Input: dimensioned drawing with shaded views. Units: mm. Origin: part minimum x, y, z. A direction names the side the tool comes from. Round coordinates to 2 decimals unless told otherwise and drop trailing zeros. Write each loop counter-clockwise with the first axis right and the second up, starting at its lowest first coordinate (ties: lowest second). Pieces come first, ordered by that corner, then holes. Notation, with made-up numbers: (68.25, 88) -> (100.25, 88) arc R18 cw to (100.25, 99) -> close; hole circle Ø10 at (43.25, 73). An arc over 180 degrees is marked (long way). One line per item, written item: value. Start each with the question number.
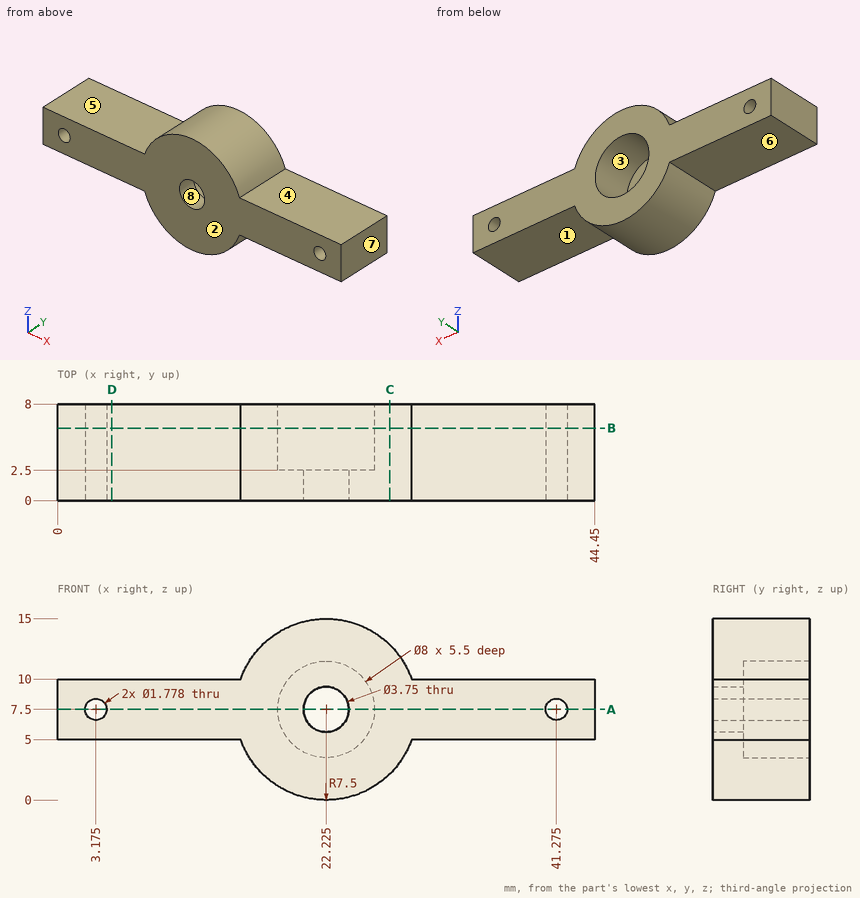
(1) Line query: probe 1 along X at (y, z) = (5.45, 7.5) (3 decimals); probe 2 along X at (y, z) = (1.5, 7.75); probe 3 along Z at (x, y) = (40, 6.5). Output: solid intervals per line, ascending.
(2) Section query D-D (x = 4.5). Output: boundary loops of the cut face in (y, z).
(3) Pull-direction query (X, two-part tool) for the marked faces 6, 7 and 8; classes: pulls with the +X half, pulls with the -X half, needs draft (parallel to the pull), parting line crosses it, or undercut.
(4) Section query B-B (y = 6). Output: boundary loops of the cut face in (x, z) (3 decimals), and give its area (3 significant figures).
(5) Section query C-C (x = 27.5). Output: boundary loops of the cut face in (y, z).
(6) Section query A-A (z = 7.5). Output: boundary loops of the cut face in (x, y) (3 decimals).
(7) Set-up query: the marked faces 1, 2, 3, 4 and 5. Return all of +Z, -Z, +X, -X, +Y, -Y with unobstructed straight access to the full face (end or side cutting, diameter ignored); none if empty.
(8) Pin query (flat end, axial travel): pin 1 (5 mm diameter, centred on x = 21, z = 8, fed in from +Y); pin 2 (2.5 mm diameter, centred on x = 8.5, y = 3, fed in from -Z); pin 3 (1.6 mm diameter, centred on x = 41.275, z = 7.5, fed in from +Y); pin 4 (4 mm diameter, centred on x = 5, y = 5.5, fed in from +Z). Return the tip coordinate at first contact, or that it passes through.
Results list:
1. probe 1: x = 0 to 2.286, 4.064 to 18.225, 26.225 to 40.386, 42.164 to 44.45
1. probe 2: x = 0 to 2.32, 4.03 to 20.37, 24.08 to 40.42, 42.13 to 44.45
1. probe 3: z = 5 to 10
2. outline: (0, 5) -> (8, 5) -> (8, 10) -> (0, 10) -> close
3. face 6: needs draft
3. face 7: pulls with the +X half
3. face 8: undercut
4. outline: (0, 5) -> (15.154, 5) arc R7.5 ccw to (29.296, 5) -> (44.45, 5) -> (44.45, 10) -> (29.296, 10) arc R7.5 ccw to (15.154, 10) -> (0, 10) -> close; hole circle Ø1.778 at (3.175, 7.5); hole circle Ø8 at (22.225, 7.5); hole circle Ø1.778 at (41.275, 7.5)
4. area: 270 mm^2
5. outline: (0, 2.17) -> (8, 2.17) -> (8, 12.83) -> (0, 12.83) -> close
6. outline: (0, 0) -> (2.286, 0) -> (2.286, 8) -> (0, 8) -> close; (4.064, 0) -> (20.35, 0) -> (20.35, 2.5) -> (18.225, 2.5) -> (18.225, 8) -> (4.064, 8) -> close; (24.1, 0) -> (40.386, 0) -> (40.386, 8) -> (26.225, 8) -> (26.225, 2.5) -> (24.1, 2.5) -> close; (42.164, 0) -> (44.45, 0) -> (44.45, 8) -> (42.164, 8) -> close
7. face 1: -Z, +X, +Y, -Y
7. face 2: +Z, -Z, +X, -X, -Y
7. face 3: +Y
7. face 4: +Z, +X, +Y, -Y
7. face 5: +Z, -X, +Y, -Y
8. pin 1: stops at y = 2.5
8. pin 2: stops at z = 5
8. pin 3: passes through
8. pin 4: stops at z = 10
